Design review of the part built by this model. Coordinates are the model's own, in mm. Face numbers are marked on the shaded views. A direction names the side the tool comes from. Give positions to 0.01 mm unless a question says otherwise; leave off trailing zeros. Order: outer loops, then holes, each group sorted by start corner. A loop starts at its lowest first (then second) coordinate and runs counter-clockwise, first axis right, second up. Notation, with made-up numbers: (41.25, 10) -> (57.25, 10) arc R16 cw to (57.25, 40) -> close; hole circle Ø6 at (-24, 65). An arc over 180 degrees is marked (long way). One line per item, written item: value. Start each with the question number.
1) Consider section A-A (z = -0.6). State the section outline as (x, y) points, plus the area to 3 significant figures.
2) For pin 1 (0.8 mm diameter, centred on x = 0, z = 2.5, fed in from -Y); pin 2 (1.1 mm diameter, centred on y = -0.5, z = 2.5, fed in from -X); pin 3 (2 mm diameter, centred on x = -1, y = -2, fed in from -Z), all flat-tipped, find the tip position at first contact; note any pin that passes through.
3) Consider section B-B (y = 4.25). State the section outline as (x, z) points, plus the area to 3 significant figures.
4) Consider section C-C (x = 5). State the section outline as (y, z) points, plus the area to 3 significant figures.
5) The part is to be moulded in two halves that separate along X. For the marked faces 3 and 4, say which applies: released by +X, released by -X, zero draft, split by the parting line, or undercut.
6) Tool access review of the marked faces 1 and 2: name each direction out of +Z, -Z, +X, -X, +Y, -Y from which nothing blocks a thin tool from reaching the whole face with its end or side.
7) Wall thickness on line 1 along X through (y, z) = (-1.5, 2.3); line 2 along X through (y, z) = (-7, 2.6); line 3 along Z through (x, y) = (2.75, -6.25): over which ranges is each line inside the solid? List them lowest first. Write a range as from..to.
from build123d import *

# Parameters (mm, degrees)
SKETCH1_W           = 12
SKETCH1_H           = 16
BOSS_EXTRUDE1_DEPTH = 2
SKETCH4_R           = 2
BOSS_EXTRUDE4_DEPTH = 16
BOSS_EXTRUDE5_DEPTH = 1


with BuildPart() as part:
    # Sketch1 → Boss-Extrude1 (new body)
    with BuildSketch(Plane.XY):
        Rectangle(SKETCH1_W, SKETCH1_H)
    extrude(amount=BOSS_EXTRUDE1_DEPTH)

    # Sketch4 → Boss-Extrude4 (add)
    with BuildSketch(Plane.XZ.offset(8)):
        with Locations((-6, 1)):
            Circle(SKETCH4_R)
        with Locations((6, 1)):
            Circle(SKETCH4_R)
    extrude(amount=-BOSS_EXTRUDE4_DEPTH)

    # Sketch5 → Boss-Extrude5 (add)
    with BuildSketch(Plane.XY.offset(2)):
        Polygon((-3.389443583, 1.106736913), (-2.742308167, 1.106736913), (-2.742308167, -2.393263087), (-3.056410731, -2.393263087), (-3.056410731, 0.747762554), (-3.594872269, 0.747762554), align=None)
        with BuildLine():
            Line((-0.992308167, 0.029813837), (-1.306410731, 0.029813837))
            add(Edge.make_bspline(
                [(-1.306410731, 0.029813837), (-1.304363578, 0.071484724), (-1.300343024, 0.153325239), (-1.281514735, 0.272649145), (-1.254573857, 0.386703944), (-1.216482403, 0.494573858), (-1.169176126, 0.597212665), (-1.112446098, 0.694212681), (-1.045252248, 0.78520387), (-0.969045514, 0.869342713), (-0.886276875, 0.946530284), (-0.796970935, 1.013185526), (-0.703125908, 1.069503198), (-0.605026509, 1.11658444), (-0.501565945, 1.151924286), (-0.393683087, 1.178145925), (-0.280903951, 1.193922271), (-0.204063929, 1.195618057), (-0.164984449, 1.196480503)],
                knots=[0, 0, 0, 0, 0.000125083, 0.00024566, 0.000361805, 0.000476223, 0.000588214, 0.000700404, 0.000812728, 0.00092691, 0.001040529, 0.001151727, 0.001260545, 0.001368429, 0.001477521, 0.001587884, 0.001701119, 0.00181831, 0.00181831, 0.00181831, 0.00181831], degree=3))
            add(Edge.make_bspline(
                [(-0.164984449, 1.196480503), (-0.126606375, 1.195582047), (-0.05119483, 1.193816612), (0.058867184, 1.178655583), (0.163644479, 1.154909991), (0.262932245, 1.121594575), (0.35593831, 1.076810147), (0.443361354, 1.023012609), (0.526242165, 0.960792777), (0.600848949, 0.887538964), (0.669357028, 0.809336579), (0.728459283, 0.725848676), (0.779072447, 0.63961939), (0.821260127, 0.549991188), (0.852316266, 0.45612016), (0.875894474, 0.359372957), (0.889221887, 0.258748146), (0.891267311, 0.190641591), (0.892307218, 0.15601576)],
                knots=[0, 0, 0, 0, 0.000115089, 0.000226145, 0.000332614, 0.000437044, 0.000539592, 0.000641561, 0.000744629, 0.00084975, 0.000954621, 0.001056175, 0.001156101, 0.001254284, 0.001352726, 0.001452208, 0.001552655, 0.001656537, 0.001656537, 0.001656537, 0.001656537], degree=3))
            add(Edge.make_bspline(
                [(0.892307218, 0.15601576), (0.890613955, 0.107267925), (0.887257144, 0.010627711), (0.858542767, -0.131387151), (0.813696256, -0.26898057), (0.759698899, -0.379717873), (0.705226455, -0.468951366), (0.656138947, -0.542420071), (0.598674136, -0.62152554), (0.531995638, -0.706002877), (0.457482766, -0.796513782), (0.374460603, -0.893003578), (0.282337121, -0.994475347), (0.21767862, -1.063780949), (0.184174205, -1.099693375)],
                knots=[0, 0, 0, 0, 0.000146118, 0.000289672, 0.0004329, 0.00057934, 0.000657978, 0.000746456, 0.000844345, 0.000951219, 0.001069268, 0.00119604, 0.001333047, 0.001480391, 0.001480391, 0.001480391, 0.001480391], degree=3))
            Line((0.184174205, -1.099693375), (-0.691526917, -2.034288728))
            Line((-0.691526917, -2.034288728), (0.937179013, -2.034288728))
            Line((0.937179013, -2.034288728), (0.937179013, -2.393263087))
            Line((0.937179013, -2.393263087), (-1.441026116, -2.393263087))
            Line((-1.441026116, -2.393263087), (-0.083654321, -0.944745458))
            add(Edge.make_bspline(
                [(-0.083654321, -0.944745458), (-0.050606434, -0.910247152), (0.012871793, -0.843982965), (0.10265437, -0.747240005), (0.183293358, -0.657490464), (0.255310751, -0.574903916), (0.317144257, -0.498272348), (0.372016488, -0.430077645), (0.415982079, -0.367323194), (0.463697475, -0.29458258), (0.509911457, -0.205770263), (0.549623813, -0.097236574), (0.573838661, 0.014490679), (0.576743497, 0.089992716), (0.578204654, 0.127970888)],
                knots=[0, 0, 0, 0, 0.000143319, 0.000275286, 0.00039593, 0.000505287, 0.000603949, 0.000691331, 0.000767782, 0.00083371, 0.000952247, 0.001067137, 0.001179618, 0.001293462, 0.001293462, 0.001293462, 0.001293462], degree=3))
            add(Edge.make_bspline(
                [(0.578204654, 0.127970888), (0.577568911, 0.151852286), (0.576315985, 0.198917937), (0.565258288, 0.267923696), (0.548547782, 0.334488509), (0.524602524, 0.398817129), (0.492995784, 0.460262781), (0.454522404, 0.518900261), (0.41013234, 0.575589226), (0.358781071, 0.628742524), (0.302369551, 0.67742373), (0.242775302, 0.720547815), (0.179725197, 0.756586926), (0.113485075, 0.786130423), (0.044239606, 0.809305804), (-0.028145139, 0.825364384), (-0.103469156, 0.835446867), (-0.154902651, 0.836811039), (-0.18111025, 0.837506144)],
                knots=[0, 0, 0, 0, 7.16e-05, 0.00014111, 0.00020913, 0.00027724, 0.000346538, 0.000415963, 0.000487357, 0.000562233, 0.000637292, 0.000710646, 0.000782564, 0.000854749, 0.000927915, 0.001001225, 0.001076884, 0.001155488, 0.001155488, 0.001155488, 0.001155488], degree=3))
            add(Edge.make_bspline(
                [(-0.18111025, 0.837506144), (-0.208481083, 0.836791112), (-0.262232879, 0.835386907), (-0.341151912, 0.825564243), (-0.41643769, 0.808618402), (-0.488279593, 0.785441728), (-0.556799178, 0.755983179), (-0.621663222, 0.719291434), (-0.682726112, 0.675507941), (-0.740102635, 0.625867385), (-0.792966614, 0.570599784), (-0.83941349, 0.508989821), (-0.879997504, 0.442162405), (-0.915406738, 0.370297855), (-0.944162428, 0.292744075), (-0.966135578, 0.20977637), (-0.983522425, 0.121754988), (-0.989330945, 0.060969904), (-0.992308167, 0.029813837)],
                knots=[0, 0, 0, 0, 8.2106e-05, 0.000161243, 0.000238127, 0.000313291, 0.000387401, 0.000461495, 0.000536397, 0.000612445, 0.000688819, 0.000765383, 0.000843422, 0.000923066, 0.001005373, 0.001091093, 0.001180334, 0.001274175, 0.001274175, 0.001274175, 0.001274175], degree=3))
        make_face()
    extrude(amount=BOSS_EXTRUDE5_DEPTH)


solid = part.part
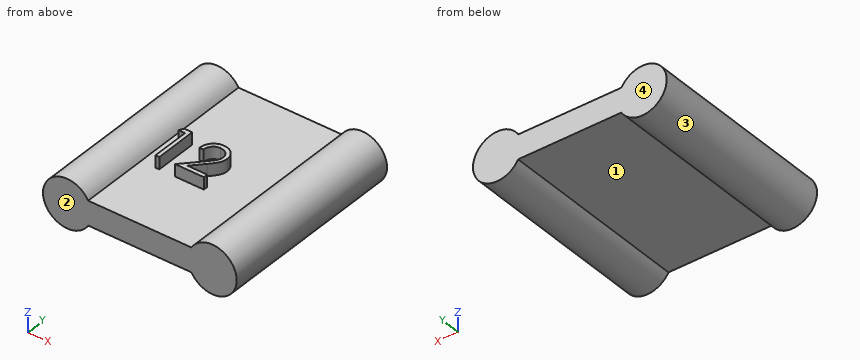
Checked values:
1. outline: (-7.2, -8) -> (-4.8, -8) -> (-4.8, 8) -> (-7.2, 8) -> close; (4.8, -8) -> (7.2, -8) -> (7.2, 8) -> (4.8, 8) -> close
1. area: 76.8 mm^2
2. pin 1: stops at y = -2.39
2. pin 2: stops at x = -7.76
2. pin 3: stops at z = 0
3. outline: (-4.27, 0) -> (4.27, 0) arc R2 ccw (long way) to (4.27, 2) -> (-4.27, 2) arc R2 ccw (long way) to start
3. area: 41.5 mm^2
4. outline: (-8, -0.73) -> (8, -0.73) -> (8, 2.73) -> (-8, 2.73) -> close
4. area: 55.4 mm^2
5. face 3: undercut
5. face 4: zero draft
6. face 1: -Z, +Y, -Y
6. face 2: +Z, -Z, +X, -X, -Y
7. line 1: x = -7.52..-4.48, -3.06..-2.74, -0.6..-0.19, 4.48..7.52
7. line 2: x = -7.2..-4.8, 4.8..7.2
7. line 3: z = 0..2
